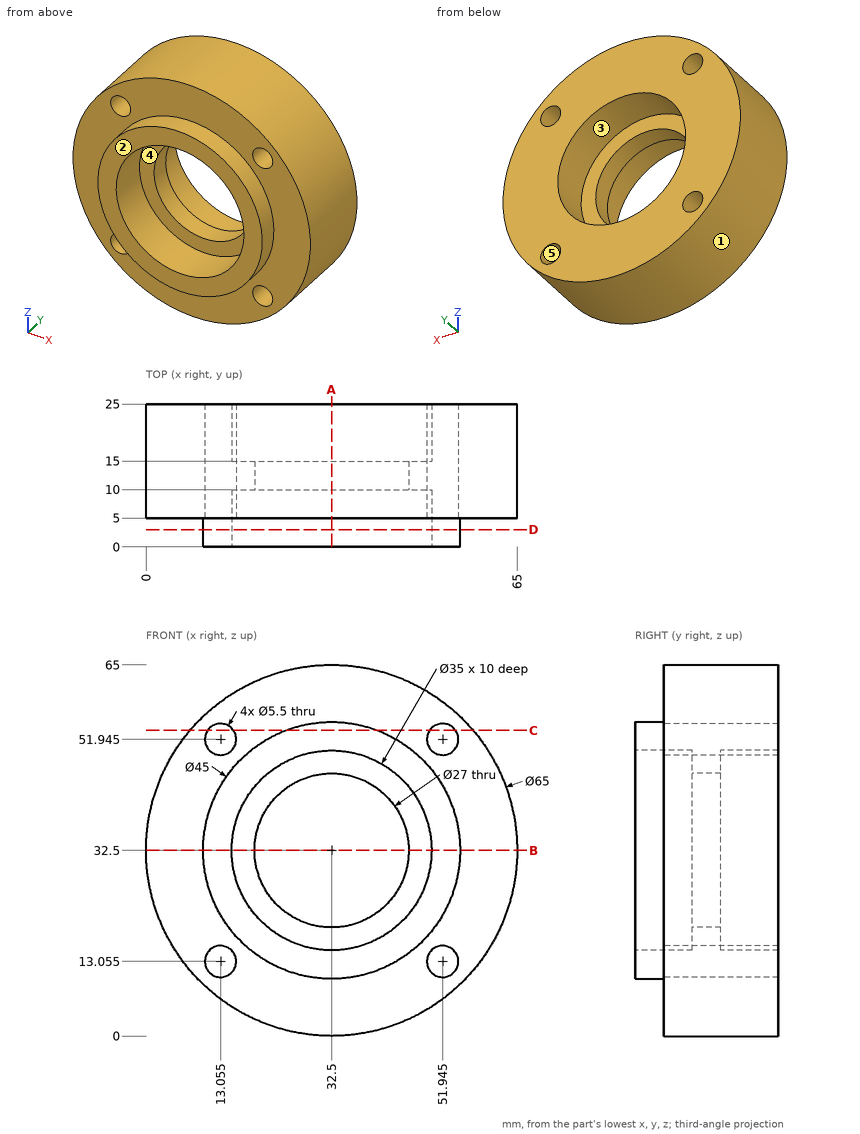
Study the drawing (mm; zero at the part's minimum x, y, z) and answer. A direction names the side the tool comes from. Give positions to 0.01 mm unless a question says otherwise; leave off trailing zeros. Order: outer loops, then holes, each group sorted by start corner. A loop starts at its lowest first (then second) coordinate and runs counter-clockwise, first axis right, second up. Notation, with made-up numbers: (-29, -22.5) - (-23, -22.5) arc R20 cw to (-23, 0.5) - close; hole circle Ø7 at (-20.5, 44). An arc over 180 degrees is marked (long way). Answer as CSV lines item,"result". Start each with the question number.
Q1. Given pin 1 Ø8 at (y, z) = (3, 24.5) entering from -X; pin 2 Ø5 at (x, y) = (52, 3) entering from +Z; pin 3 Ø6 at (y, z) = (14, 47.5) entering from +X, each flat-ended and moving along its own axis, determine where each tip first touches the part or whether it passes through.
Q2. The part is cut by section B-B (z = 32.5). Write down the section's boundary in (x, y).
Q3. The part is cut by section D-D (y = 3). Write down the section's boundary in (x, z).
Q4. Find the intervals of material crossed by L1, parallel to X at y = 13.25, z = 32.5; L2, parallel to Z at x = 15.5, y = 12 (1 decimal); L3, parallel to Z at x = 12.5, y = 22.5, in increasing order. Write a range as [from, to].
Q5. The part is cut by section C-C (z = 53.5). Write down the section's boundary in (x, y) (1 decimal).
Q6. The mould has two halves that part along X. Classify the marked faces 1, 2 and 3: +X half, -X half, draft (parallel to the pull), parting line (faces both ways), or undercut.
Q7. The part is cut by section A-A (x = 32.5). Write down the section's boundary in (y, z).
Q8. For the marked faces 4 and 5, determine the directions among +Z, -Z, +X, -X, +Y, -Y from which every point of the face is accessible in a straight line to the end or side of a thin tool.
Check result:
1,pin 1,"stops at x = 0.32"
1,pin 2,"stops at z = 59.56"
1,pin 3,"stops at x = 62.7"
2,outline,"(0, 5) - (10, 5) - (10, 0) - (15, 0) - (15, 10) - (19, 10) - (19, 15) - (15, 15) - (15, 25) - (0, 25) - close; (46, 10) - (50, 10) - (50, 0) - (55, 0) - (55, 5) - (65, 5) - (65, 25) - (50, 25) - (50, 15) - (46, 15) - close"
3,outline,"circle Ø45 at (32.5, 32.5); hole circle Ø35 at (32.5, 32.5)"
4,L1,"x = [0, 19], [46, 65]"
4,L2,"z = [4.8, 11.8], [14.3, 50.7], [53.2, 60.2]"
4,L3,"z = [6.88, 10.36], [15.75, 49.25], [54.64, 58.12]"
5,outline,"(7.7, 5) - (10.8, 5) - (10.8, 25) - (7.7, 25) - close; (15.3, 5) - (24.4, 5) - (24.4, 0) - (40.6, 0) - (40.6, 5) - (49.7, 5) - (49.7, 25) - (15.3, 25) - close; (54.2, 5) - (57.3, 5) - (57.3, 25) - (54.2, 25) - close"
6,face 1,"parting line"
6,face 2,"draft"
6,face 3,"undercut"
7,outline,"(0, 10) - (5, 10) - (5, 0) - (25, 0) - (25, 15) - (15, 15) - (15, 19) - (10, 19) - (10, 15) - (0, 15) - close; (0, 50) - (10, 50) - (10, 46) - (15, 46) - (15, 50) - (25, 50) - (25, 65) - (5, 65) - (5, 55) - (0, 55) - close"
8,face 4,"-Y"
8,face 5,"+Y, -Y"
